Geometry: final body of the model. Coordinates: model frame, mm. Give positions to 0.01 mm unless a question says otherwise; leave off trailing zeros. Order: outer loops, then holes, each group sorted by start corner. A loop starts at its lowest first (then second) coordinate and runs counter-clockwise, first axis right, second up. Notation, with made-up numbers: (5.5, 25) -> (13.5, 25) arc R20 ccw to (13.5, 64) -> close; hole circle Ø3 at (23, -3.75). An arc over 180 degrees is marked (long way). Write item = value, one per line.
Autodesk Inventor part; units mm, degrees
ref_plane "YZ Plane" through (0, 0, 0) normal (1, 0, 0) x (0, 1, 0)
ref_plane "XZ Plane" through (0, 0, 0) normal (0, 1, 0) x (-1, 0, 0)
ref_plane "XY Plane" through (0, 0, 0) normal (0, 0, 1) x (1, 0, 0)
sketch "Sketch2" plane through (0, 0, 0) normal (0, 0, 1) x (1, 0, 0)
  line L0 (-103, 103) -> (103, 103)
  line L1 (103, 103) -> (103, -103)
  line L2 (103, -103) -> (-103, -103)
  line L3 (-103, -103) -> (-103, 103)
  line L4 (-103, 103) -> (103, -103) construction
  line L5 (103, 103) -> (-103, -103) construction
  line L6 (-103, 103) -> (-98, 103)
  line L7 (-98, 103) -> (-98, 98)
  line L8 (-98, 98) -> (-103, 98)
  line L9 (-103, 98) -> (-103, 103)
  line L10 (103, 103) -> (98, 103)
  line L11 (98, 103) -> (98, 98)
  line L12 (98, 98) -> (103, 98)
  line L13 (103, 98) -> (103, 103)
  line L14 (103, -103) -> (98, -103)
  line L15 (98, -103) -> (98, -98)
  line L16 (98, -98) -> (103, -98)
  line L17 (103, -98) -> (103, -103)
  line L18 (-103, -103) -> (-98, -103)
  line L19 (-98, -103) -> (-98, -98)
  line L20 (-98, -98) -> (-103, -98)
  line L21 (-103, -98) -> (-103, -103)
  line L22 (90, 89) -> (90, -89)
  line L23 (-90, 90) -> (90, -90) construction
  line L24 (90, 90) -> (-90, -90) construction
  line L25 (-91, 90) -> (-96, 90)
  line L26 (-97, 89) -> (-97, -89)
  line L27 (-96, -90) -> (-91, -90)
  line L28 (-90, -89) -> (-90, 89)
  line L29 (91, 90) -> (96, 90)
  line L30 (97, 89) -> (97, -89)
  line L31 (96, -90) -> (91, -90)
  arc A0 (-96, 90) -> (-97, 89) centre (-96, 89) ccw
  arc A1 (-90, 89) -> (-91, 90) centre (-91, 89) ccw
  arc A2 (-91, -90) -> (-90, -89) centre (-91, -89) ccw
  arc A3 (-97, -89) -> (-96, -90) centre (-96, -89) ccw
  arc A4 (97, 89) -> (96, 90) centre (96, 89) ccw
  arc A5 (91, 90) -> (90, 89) centre (91, 89) ccw
  arc A6 (96, -90) -> (97, -89) centre (96, -89) ccw
  arc A7 (90, -89) -> (91, -90) centre (91, -89) ccw
  point P0 (0, 0)
  point P1 (-97, -90)
  point P2 (97, -90)
  dimension "d0" = 206
  dimension "d1" = 206
  dimension "d2" = 5
  dimension "d3" = 5
  dimension "d4" = 5
  dimension "d5" = 5
  dimension "d6" = 5
  dimension "d7" = 5
  dimension "d8" = 5
  dimension "d9" = 5
  dimension "d10" = 180
  dimension "d11" = 180
  dimension "d12" = 7
  dimension "d14" = 1
  dimension "d15" = 180
extrude "Extrusion1" add sketch "Sketch2" along normal blind 2 contours L0 L11 L12 L1 L16 L15 L2 L19 L20 L3 L8 L7
sketch "Sketch3" plane through (0, 0, 2) normal (0, 0, 1) x (1, 0, 0)
  circle A0 centre (-85, 86.25) radius 1.825
  point P0 (0, 0)
  dimension "d18" = 3.65
hole "Hole1" at (-85, 86.25, 2) direction (0, 0, -1) diameter 3.6 depth 10
pattern_linear "Rectangular Pattern1" count 2 spacing 80 along (1, 0, 0) count 6 spacing 30 along (0, -1, 0) of "Hole1"
sketch "Sketch4" plane through (0, 0, 2) normal (0, 0, 1) x (1, 0, 0)
  circle A0 centre (5, 63.75) radius 1.8
  line L0 (98, 103) -> (-98, 103)
  point P0 (0, 0)
  dimension "d33" = 3.6
  dimension "d47" = 39.25
hole "Hole2" at (5, 63.75, 2) direction (0, 0, -1) diameter 3.6 depth 10
pattern_linear "Rectangular Pattern2" count 2 spacing 80 along (1, 0, 0) count 6 spacing 30 along (0, -1, 0) of "Hole2"
properties part number "Baseplate_for_PCBs_mirroredHoles"
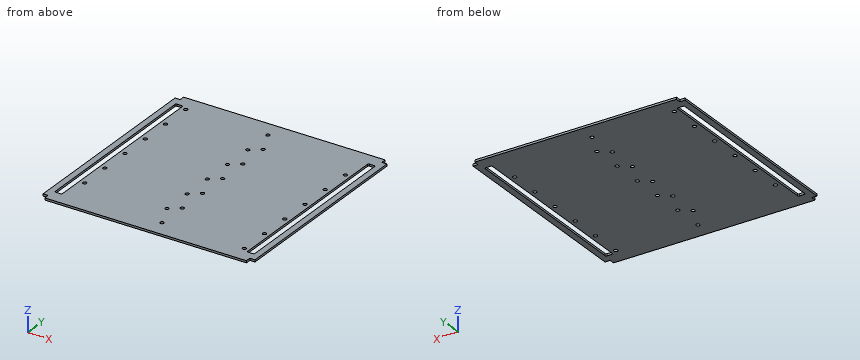
1) Section query A-A (y = 69.5). Output: boundary loops of the cut face in (x, z), plus the area to 3 significant figures.
Check sheet entries:
outline = (-103, 0) -> (-97, 0) -> (-97, 2) -> (-103, 2) -> close; (-90, 0) -> (90, 0) -> (90, 2) -> (-90, 2) -> close; (97, 0) -> (103, 0) -> (103, 2) -> (97, 2) -> close
area = 384 mm²
2) Line query: line 1 (X direction, y = -22, z = 1.5); line 2 (X direction, y = -33.75, z = 1.1); line 3 (X direction, y = -86.25, z = 1.3). Output: solid intervals per line, ascending. Write a range as from..to.
Check sheet entries:
line_1 = -103..-97, -90..90, 97..103
line_2 = -103..-97, -90..-86.8, -83.2..-6.8, -3.2..90, 97..103
line_3 = -103..-97, -90..3.2, 6.8..83.2, 86.8..90, 97..103
3) Section query B-B (z = 1.2). Count the separate pieces of the cut face and the enclosed holes in it, plus the area to 3 significant figures.
Check sheet entries:
separate_pieces = 1
enclosed_holes = 26
area = 39,600 mm²
4) First-contact query: P1, Ø3, axis at x = -85, y = 26.25, coming from the +Z side. Flat tip, straight axial feed; report the tip coordinate or a pass-through.
Check sheet entries:
P1 = through
